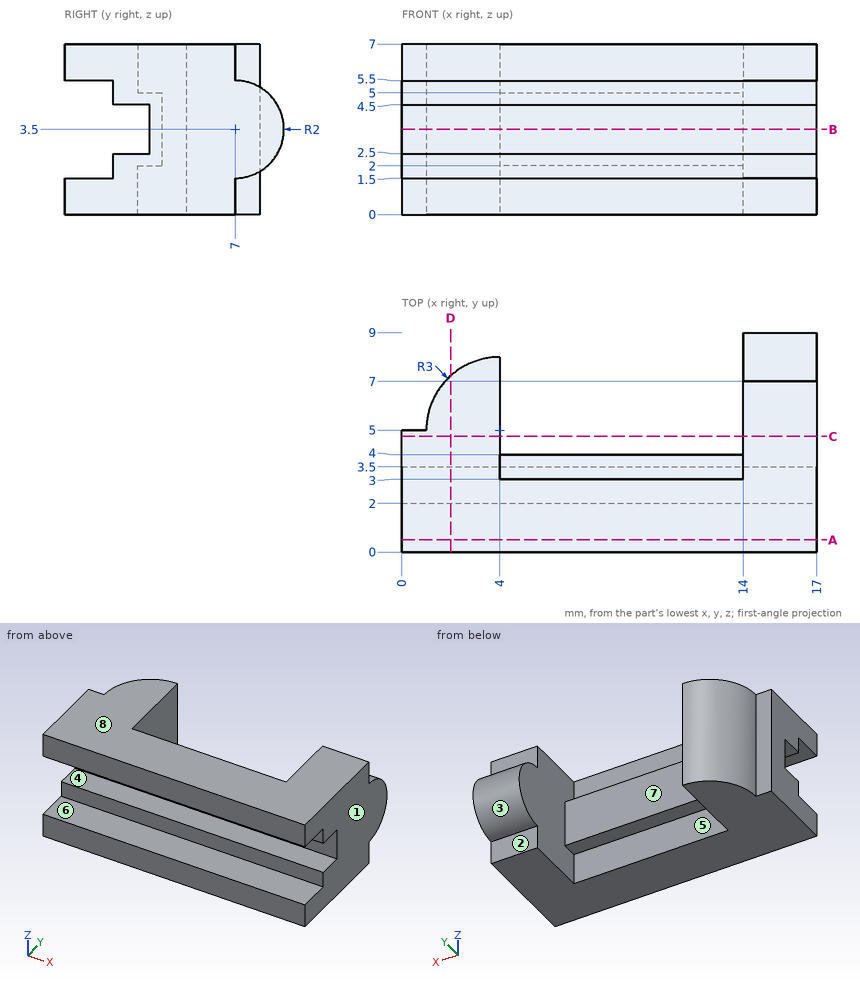
Geometry: see drawing. Coordinates: mm, zero at the bounding-box minimum. A direction names the side the tool comes from. Round coordinates to 2 decimals unless told otherwise and drop trailing zeros. Loops run counter-clockwise (first coordinate to the right, second up) from the corner with the lowest first, then second, coordinate; pieces in that order, holes last. Notation, with made-up numbers: M 29.5,24 L 43.5,24 A16 cw 43.5,37 Z; hole C 18.5,65 d5. An arc over 180 degrees is marked long. Use a Markdown table: item, result. Add a question column.
1. Section query B-B on z = 3.5. Return the cut outline in (x, y).
2. Section query D-D on x = 2. Return the cut outline in (y, z), then the cut area to 3 significant figures.
3. Contact query for flat-ended pins moving along their axis: P1, Ø0.8, axis at x = 11, y = 3.5, coming from the -Z side; P2, Ø1.6, axis at x = 12.5, y = 1, coming from the -Z side; P3, Ø0.8, axis at x = 10, z = 2, coming from the -Y side; P4, Ø0.6, axis at x = 8.5, z = 6, coming from the +Y side. Output: stop coordinate, or through.
4. Line query: line 1 (X direction, y = 4.5, z = 5); line 2 (Z direction, x = 12, y = 0.75); line 3 (Z direction, x = 1.75, y = 2.25). Output: solid intervals per line, ascending.
5. Reachability of the marked faces 1, 2, 3, 4 and 5 from +Z, -Z, +X, -X, +Y, -Y: full face, straight path, thin tool, end or side. Return the list, or none.
6. Section query A-A on y = 0.5. Return the cut outline in (x, z).
7. Section query C-C on y = 4.75. Return the cut outline in (x, z).
8. Mould query, pull axis Z, two halves, no side actions, for the marked faces 6, 7 and 8. Classes: pulls with the +Z half, pulls with the -Z half, needs draft (parallel to the pull), parting line crosses it, or undercut.
Reported:
| question | item | result |
|---|---|---|
| 1 | outline | M 0,3.5 L 17,3.5 L 17,9 L 14,9 L 14,4 L 4,4 L 4,8 A3 ccw 1,5 L 0,5 Z |
| 2 | outline | M 0,0 L 7.24,0 L 7.24,7 L 0,7 L 0,5.5 L 2,5.5 L 2,4.5 L 3.5,4.5 L 3.5,2.5 L 2,2.5 L 2,1.5 L 0,1.5 Z |
| 2 | area | 39.7 mm² |
| 3 | P1 | stops at z = 2 |
| 3 | P2 | stops at z = 0 |
| 3 | P3 | stops at y = 2 |
| 3 | P4 | stops at y = 3 |
| 4 | line 1 | x = 0 to 4, 14 to 17 |
| 4 | line 2 | z = 0 to 1.5, 5.5 to 7 |
| 4 | line 3 | z = 0 to 2.5, 4.5 to 7 |
| 5 | face 1 | +Z, -Z, +X, +Y, -Y |
| 5 | face 2 | -Z, +X, +Y |
| 5 | face 3 | +X, +Y |
| 5 | face 4 | +X, -X, -Y |
| 5 | face 5 | -Z, +Y |
| 6 | outline | M 0,0 L 17,0 L 17,1.5 L 0,1.5 Z; M 0,5.5 L 17,5.5 L 17,7 L 0,7 Z |
| 7 | outline | M 0,0 L 4,0 L 4,7 L 0,7 Z; M 14,0 L 17,0 L 17,7 L 14,7 Z |
| 8 | face 6 | undercut |
| 8 | face 7 | needs draft |
| 8 | face 8 | pulls with the +Z half |
